Model file for the job. Use its own axes, mm. A direction names the side the tool comes from. Give positions to 0.01 mm unless a question says otherwise; leave off trailing zeros. Loops run counter-clockwise (first coordinate to the right, second up) from the corner with the lowest first, then second, coordinate; pieces in that order, holes last. Notation, with made-up numbers: M 76.5,-31 L 89.5,-31 A8 cw 89.5,-19 Z; hole C 83.5,79 d9. An arc over 180 degrees is marked long. Use CSV: the item, a comma, the result in double quotes. Start each with the question number.
(1) Slice it at B-B on x = -9. List the corners of the cut face in (y, z).
(2) Slice it at A-A on x = 4. List the corners of the cut face in (y, z) (3 decimals).
(3) Flat gauge pins, fed straight in: P1, Ø6, axis at x = -16, y = -6, coming from the -Z side; P2, Ø10, axis at x = -55, z = -8.5, coming from the -Y side; P3, Ø2.5, axis at y = -1.98, z = 9.29, coming from the -X side. Where does each tip first touch, or does it go through?
(4) Wall check: line 1 along Z through (x, y) = (-60.5, 11); line 2 along X through (y, z) = (-0.5, -11); line 3 along Y through (x, z) = (3.5, -14.5). Give the ranges that are in metal, low to high. Write a range as from..to.
(5) Tool access for faces 4 (the face through (-65.05, 3, -3)), 5 (the face through (-68, 0, 12.7)), 6 (the face through (4.87, -8.06, -6.58)): list every direction of +Z, -Z, +X, -X, +Y, -Y with a clear straight run to the whole face (end or side of a thin tool).
(6) Two-plate mould, pull along Z, no slides. Class faces 1 (the face through (10.6, -3.3, 0.1)), 2 (the face through (-30.273, -10.648, 13.887)), 3 (the face through (2.291, 9.185, -3.031)): pulls with the +Z half, pulls with the -Z half, needs draft (parallel to the pull), parting line crosses it, or undercut.
```python
from build123d import *

# Parameters (mm, degrees)
SKETCH1_R                          = 17.5
BOSS_EXTRUDE1_DEPTH                = 61.5
SKETCH3_R                          = 17.3
BOSS_EXTRUDE2_DEPTH                = 7.3
SKETCH4_R                          = 6.5
BOSS_EXTRUDE3_DEPTH                = 1.1
SKETCH5_R                          = 5
BOSS_EXTRUDE4_DEPTH                = 2.2
SKETCH6_R                          = 3
BOSS_EXTRUDE5_DEPTH                = 16.7
SKETCH7_R                          = 16.425
BOSS_EXTRUDE6_DEPTH                = 2.2
BOSS_EXTRUDE7_START                = 1.35
SKETCH8_R                          = 6.5
BOSS_EXTRUDE7_DEPTH                = 1.35
SKETCH9_R                          = 3.5
BOSS_EXTRUDE8_DEPTH                = 2.05
SKETCH10_R                         = 2
BOSS_EXTRUDE9_DEPTH                = 12.2
BOSS_EXTRUDE10_DEPTH               = 8
CHAMFER1_SIZE                      = 0.3
CHAMFER2_SIZE                      = 0.2
CHAMFER3_SIZE                      = 1
CHAMFER4_SIZE                      = 0.8
M2_5X0_45_TAPPED_HOLE1_D           = 2.05
M2_5X0_45_TAPPED_HOLE1_DEPTH       = 4.5
M2_5X0_45_TAPPED_HOLE1_CSINK_D     = 2.65
M2_5X0_45_TAPPED_HOLE1_CSINK_ANGLE = 90
M2_5X0_45_TAPPED_HOLE1_TIP         = 0.615882135
M2X0_4_TAPPED_HOLE1_D              = 1.6
M2X0_4_TAPPED_HOLE1_DEPTH          = 3
M2X0_4_TAPPED_HOLE1_CSINK_D        = 2.1
M2X0_4_TAPPED_HOLE1_CSINK_ANGLE    = 90
M2X0_4_TAPPED_HOLE1_TIP            = 0.480688495
M1_6X0_35_TAPPED_HOLE1_D           = 1.25
M1_6X0_35_TAPPED_HOLE1_DEPTH       = 4.95
M1_6X0_35_TAPPED_HOLE1_CSINK_D     = 1.7
M1_6X0_35_TAPPED_HOLE1_CSINK_ANGLE = 90
M1_6X0_35_TAPPED_HOLE1_TIP         = 0.375537887


with BuildPart() as part:
    # Sketch1 → Boss-Extrude1 (new body)
    with BuildSketch(Plane(origin=(0, 0, 0), x_dir=(0, 0, -1), z_dir=(1, 0, 0))):
        Circle(SKETCH1_R)
    extrude(amount=-BOSS_EXTRUDE1_DEPTH)

    # Sketch3 → Boss-Extrude2 (add)
    with BuildSketch(Plane(origin=(0, 0, 0), x_dir=(0, 0, -1), z_dir=(1, 0, 0))):
        Circle(SKETCH3_R)
    extrude(amount=BOSS_EXTRUDE2_DEPTH)

    # Sketch4 → Boss-Extrude3 (add)
    with BuildSketch(Plane(origin=(7.3, 0, 0), x_dir=(0, 0, -1), z_dir=(1, 0, 0))):
        Circle(SKETCH4_R)
    extrude(amount=BOSS_EXTRUDE3_DEPTH)

    # Sketch5 → Boss-Extrude4 (add)
    with BuildSketch(Plane(origin=(8.4, 0, 0), x_dir=(0, 0, -1), z_dir=(1, 0, 0))):
        Circle(SKETCH5_R)
    extrude(amount=BOSS_EXTRUDE4_DEPTH)

    # Sketch6 → Boss-Extrude5 (add)
    with BuildSketch(Plane(origin=(10.6, 0, 0), x_dir=(0, 0, -1), z_dir=(1, 0, 0))):
        Circle(SKETCH6_R)
    extrude(amount=BOSS_EXTRUDE5_DEPTH)

    # Sketch7 → Boss-Extrude6 (add)
    with BuildSketch(Plane.ZY.offset(61.5)):
        with Locations(Location((0, 0, 0), (0, 0, 180))):
            Circle(SKETCH7_R)
    extrude(amount=BOSS_EXTRUDE6_DEPTH)

    # Sketch8 → Boss-Extrude7 (add)
    with BuildSketch(Plane.ZY.offset(63.7).offset(BOSS_EXTRUDE7_START)):
        with Locations(Location((0, 0, 0), (0, 0, 180))):
            Circle(SKETCH8_R)
    extrude(amount=-BOSS_EXTRUDE7_DEPTH)

    # Sketch9 → Boss-Extrude8 (add)
    with BuildSketch(Plane.ZY.offset(65.05)):
        Circle(SKETCH9_R)
    extrude(amount=BOSS_EXTRUDE8_DEPTH)

    # Sketch10 → Boss-Extrude9 (add)
    with BuildSketch(Plane.ZY.offset(67.1)):
        Circle(SKETCH10_R)
    extrude(amount=BOSS_EXTRUDE9_DEPTH)

    # Sketch11 → Boss-Extrude10 (add)
    with BuildSketch(Plane.ZY.offset(63.7)):
        Polygon((-12.7, 1.4), (-13.2, 1.4), (-13.2, 0), (-13.2, -1.4), (-12.7, -1.4), (-12.7, 0), align=None)
        Polygon((12.7, -1.4), (13.2, -1.4), (13.2, 0), (13.2, 1.4), (12.7, 1.4), (12.7, 0), align=None)
    extrude(amount=BOSS_EXTRUDE10_DEPTH)

    # Chamfer1
    chamfer1_edges = [part.edges().sort_by_distance(p)[0] for p in [
        (8.4, 0, 6.5),
        (27.3, 0, 3),
        (-63.7, 0, 16.425),
        (-65.05, 0, 6.5),
        (-79.3, 0, -2),
        (-61.5, 0, 17.5),
    ]]
    chamfer(chamfer1_edges, length=CHAMFER1_SIZE)

    # Chamfer2
    chamfer2_edges = [part.edges().sort_by_distance(p)[0] for p in [
        (0, 0, 17.5),
    ]]
    chamfer(chamfer2_edges, length=CHAMFER2_SIZE - 0.0001)  # a hair under: the kernel refuses the full size

    # Chamfer3
    chamfer3_edges = [part.edges().sort_by_distance(p)[0] for p in [
        (7.3, 0, 17.3),
    ]]
    chamfer(chamfer3_edges, length=CHAMFER3_SIZE)

    # Chamfer4
    chamfer4_edges = [part.edges().sort_by_distance(p)[0] for p in [
        (-71.7, 1.4, -12.95),
        (-71.7, -1.4, -12.95),
        (-71.7, -1.4, 12.95),
        (-71.7, 1.4, 12.95),
    ]]
    chamfer(chamfer4_edges, length=CHAMFER4_SIZE)

    # M2.5x0.45 Tapped Hole1
    with Locations(Plane(origin=(7.3, 0, 0), x_dir=(0, 0, -1), z_dir=(1, 0, 0))):
        with Locations((-6.35674076, 7.059875842), (2.935661447, 9.035036905), (9.292402207, 1.975161063), (6.35674076, -7.059875842), (-2.935661447, -9.035036905), (-9.292402207, -1.975161063)):
            CounterSinkHole(M2_5X0_45_TAPPED_HOLE1_D / 2, M2_5X0_45_TAPPED_HOLE1_CSINK_D / 2, depth=M2_5X0_45_TAPPED_HOLE1_DEPTH, counter_sink_angle=M2_5X0_45_TAPPED_HOLE1_CSINK_ANGLE)
            with Locations((0, 0, -(M2_5X0_45_TAPPED_HOLE1_DEPTH + M2_5X0_45_TAPPED_HOLE1_TIP / 2))):  # 118° drill point
                Cone(0, M2_5X0_45_TAPPED_HOLE1_D / 2, M2_5X0_45_TAPPED_HOLE1_TIP, mode=Mode.SUBTRACT)

    # M2x0.4 Tapped Hole1
    with Locations(Plane.ZY.offset(63.7)):
        with Locations((8.619260655, 11.03215055), (-5.244492308, 12.980573964), (-8.619260655, -11.03215055), (5.244492308, -12.980573964)):
            CounterSinkHole(M2X0_4_TAPPED_HOLE1_D / 2, M2X0_4_TAPPED_HOLE1_CSINK_D / 2, depth=M2X0_4_TAPPED_HOLE1_DEPTH, counter_sink_angle=M2X0_4_TAPPED_HOLE1_CSINK_ANGLE)
            with Locations((0, 0, -(M2X0_4_TAPPED_HOLE1_DEPTH + M2X0_4_TAPPED_HOLE1_TIP / 2))):  # 118° drill point
                Cone(0, M2X0_4_TAPPED_HOLE1_D / 2, M2X0_4_TAPPED_HOLE1_TIP, mode=Mode.SUBTRACT)

    # M1.6x0.35 Tapped Hole1
    with Locations(Plane.ZY.offset(63.7)):
        with Locations((-6.540983551, 10.886024719), (-10.886024719, -6.540983551), (6.540983551, -10.886024719), (10.886024719, 6.540983551)):
            CounterSinkHole(M1_6X0_35_TAPPED_HOLE1_D / 2, M1_6X0_35_TAPPED_HOLE1_CSINK_D / 2, depth=M1_6X0_35_TAPPED_HOLE1_DEPTH, counter_sink_angle=M1_6X0_35_TAPPED_HOLE1_CSINK_ANGLE)
            with Locations((0, 0, -(M1_6X0_35_TAPPED_HOLE1_DEPTH + M1_6X0_35_TAPPED_HOLE1_TIP / 2))):  # 118° drill point
                Cone(0, M1_6X0_35_TAPPED_HOLE1_D / 2, M1_6X0_35_TAPPED_HOLE1_TIP, mode=Mode.SUBTRACT)


solid = part.part
```
Reply:
1,outline,"C 0,0 d35"
2,outline,"C 0,0 d34.6; hole C -9.035,2.936 d2.05; hole C -7.06,-6.357 d2.05; hole C -1.975,9.292 d2.05; hole C 1.975,-9.292 d2.05; hole C 7.06,6.357 d2.05; hole C 9.035,-2.936 d2.05"
3,P1,"stops at z = -17.24"
3,P2,"stops at y = -17.15"
3,P3,"stops at x = -63.7"
4,line 1,"z = -13.61..-7.16, -5.93..8.15, 9.09..13.61"
4,line 2,"x = -63.7..7.3"
4,line 3,"y = -9.44..9.44"
5,face 4,"-X"
5,face 5,"-X, +Y, -Y"
5,face 6,"+X"
6,face 1,"needs draft"
6,face 2,"parting line crosses it"
6,face 3,"undercut"
